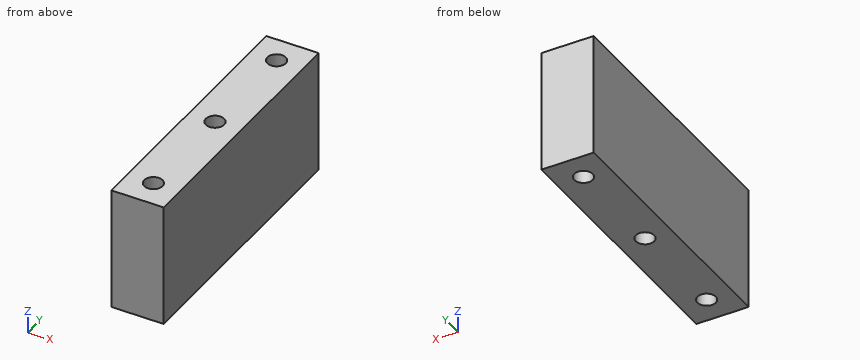
```python
from build123d import *

# Parameters (mm, degrees)
SKETCH017_W   = 8.5
SKETCH017_H   = 44
PAD001_DEPTH  = 20
SKETCH016_R   = 1.5
HOLE001_DEPTH = 4
SKETCH019_R   = 1.5
HOLE003_DEPTH = 4


with BuildPart() as part:
    # Sketch017 → Pad001 (new body)
    with BuildSketch(Plane.XY):
        with Locations((166.25, 22)):
            Rectangle(SKETCH017_W, SKETCH017_H)
    extrude(amount=PAD001_DEPTH)

    # Sketch016 → Hole001 (cut)
    with BuildSketch(Plane.XY):
        with Locations((166.244797, 39.500001)):
            Circle(SKETCH016_R)
        with Locations((166.247574, 22)):
            Circle(SKETCH016_R)
        with Locations((166.247574, 4.5)):
            Circle(SKETCH016_R)
    extrude(amount=HOLE001_DEPTH, mode=Mode.SUBTRACT)

    # Sketch019 (on Face5 of Hole001) → Hole003 (cut)
    with BuildSketch(Plane.XY.offset(20)):
        with Locations((166.244797, 39.500001)):
            Circle(SKETCH019_R)
        with Locations((166.247574, 22)):
            Circle(SKETCH019_R)
        with Locations((166.247574, 4.5)):
            Circle(SKETCH019_R)
    extrude(amount=-HOLE003_DEPTH, mode=Mode.SUBTRACT)


solid = part.part
```
Source: CAD feature listing. Evaluate the final solid. Frame: model axes, mm. Coordinates: 2 decimals unless noted, no trailing zeros. Loops run counter-clockwise (first coordinate to the right, second up) from the corner with the lowest first, then second, coordinate; pieces in that order, holes last. Notation, with made-up numbers: M 2,-6 L 10,-6 A24 cw 10,22 Z; hole C -11.75,8.25 d7. An arc over 180 degrees is marked long. Put each result on its own line as item: value. Start each with the question number.
1) Ray query, L1, parallel to Y at x = 166.5, z = 3.5; L2, parallel to Z at x = 167, y = 5. Return the intervals inside material, ascending. Write a range as from..to.
2) Contact query for flat-ended pins moving along their axis: pin 1 Ø0.9 at (x, y) = (166, 4.5) entering from -Z; pin 2 Ø2.5 at (x, y) = (166.25, 4.5) entering from +Z. Output: stop coordinate, or through.
3) Cut plane B-B on y = 39.5. Return the cut outline in (x, z).
4) Cut plane A-A on z = 2.75. Return the cut outline in (x, y), then the cut area to 3 significant figures.
The answers:
1. L1: y = 0..3.02, 5.98..20.52, 23.48..38.02, 40.98..44
1. L2: z = 4..16
2. pin 1: stops at z = 4
2. pin 2: stops at z = 16
3. outline: M 162,0 L 164.74,0 L 164.74,4 L 167.74,4 L 167.74,0 L 170.5,0 L 170.5,20 L 167.74,20 L 167.74,16 L 164.74,16 L 164.74,20 L 162,20 Z
4. outline: M 162,0 L 170.5,0 L 170.5,44 L 162,44 Z; hole C 166.24,39.5 d3; hole C 166.25,4.5 d3; hole C 166.25,22 d3
4. area: 353 mm²
